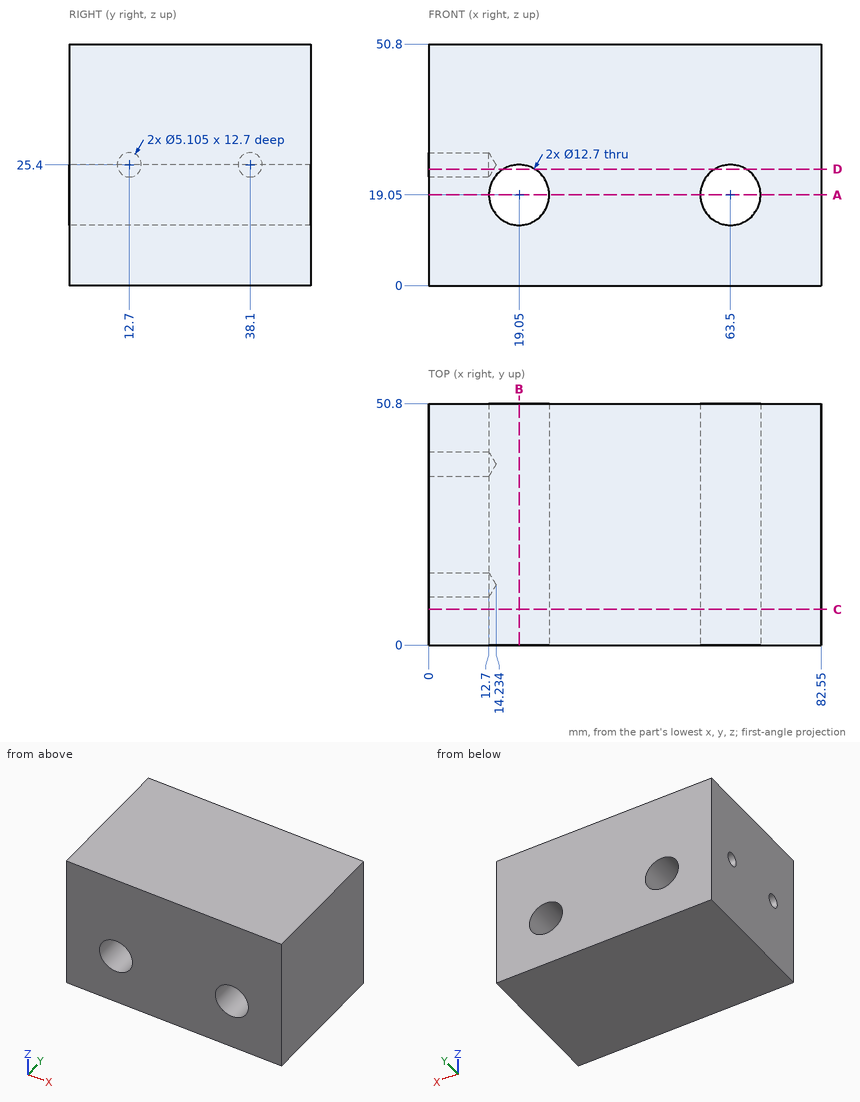
Design review of the part shown in the three views and the two pictorial views. Dimensions are in mm from the part's minimum x, y and z. Give positions to 0.01 mm unless a question says otherwise; leave off trailing zeros. Loops run counter-clockwise (first coordinate to the right, second up) from the corner with the lowest first, then second, coordinate; pieces in that order, holes last. Notation, with made-up numbers: (51, -26.5) -> (63, -26.5) arc R23 ccw to (63, -12.5) -> close; hole circle Ø5 at (86, -17). An arc over 180 degrees is marked (long way). One line per item, written item: value.
Q1. For L1, parallel to Y at x = 3, z = 25.4; L2, parallel to X at y = 13.5, z = 19.05; L3, parallel to Z at x = 19.05, y = 22.5, list the stretches that pass through material, from the lowest coordinate up.
Numbers:
L1: y = 0 to 10.15, 15.25 to 35.55, 40.65 to 50.8
L2: x = 0 to 12.7, 25.4 to 57.15, 69.85 to 82.55
L3: z = 0 to 12.7, 25.4 to 50.8
Q2. We need section D-D on z = 24.5. Give the number of separate pieces and of enclosed holes in the cut face, and give its area (3 significant figures).
Numbers:
separate pieces: 3
enclosed holes: 0
area: 3,400 mm^2
Q3. We need section C-C on y = 7.5. Give the boundary of the cut face in (x, z), and give its area (3 significant figures).
Numbers:
outline: (0, 0) -> (82.55, 0) -> (82.55, 50.8) -> (0, 50.8) -> close; hole circle Ø12.7 at (19.05, 19.05); hole circle Ø12.7 at (63.5, 19.05)
area: 3,940 mm^2
Q4. We need section A-A on z = 19.05. Give the boundary of the cut face in (x, y), and give its area (3 significant figures).
Numbers:
outline: (0, 0) -> (12.7, 0) -> (12.7, 50.8) -> (0, 50.8) -> close; (25.4, 0) -> (57.15, 0) -> (57.15, 50.8) -> (25.4, 50.8) -> close; (69.85, 0) -> (82.55, 0) -> (82.55, 50.8) -> (69.85, 50.8) -> close
area: 2,900 mm^2
Q5. We need section B-B on x = 19.05. Give the boundary of the cut face in (y, z).
Numbers:
outline: (0, 0) -> (50.8, 0) -> (50.8, 12.7) -> (0, 12.7) -> close; (0, 25.4) -> (50.8, 25.4) -> (50.8, 50.8) -> (0, 50.8) -> close
Q6. For pin 1 Ø4.5 at (y, z) = (12.7, 25.4) entering from -X; pin 2 Ø7.5 at (x, z) = (19.05, 19.05) entering from +Y, all flat-tipped, find the tip position at first contact; note any pin that passes through.
Numbers:
pin 1: stops at x = 12.88
pin 2: passes through
